from build123d import *

# Parameters (mm, degrees)
BOSS_EXTRUDE1_DEPTH = 5.75
SKETCH2_R           = 2.5
BOSS_EXTRUDE2_DEPTH = 10.5
BOSS_EXTRUDE3_DEPTH = 16.25
SKETCH4_R           = 5
SKETCH4_R_2         = 2.5
BOSS_EXTRUDE5_DEPTH = 8.5
SKETCH5_R           = 2.5
BOSS_EXTRUDE6_DEPTH = 16.25
BOSS_EXTRUDE7_START = 8.5
SKETCH6_R           = 5
BOSS_EXTRUDE7_DEPTH = 8.5
BOSS_EXTRUDE8_START = 8
SKETCH7_R           = 2.5
BOSS_EXTRUDE8_DEPTH = 8
SKETCH8_W           = 10.5
SKETCH8_H           = 5
CUT_EXTRUDE2_DEPTH  = 20
SKETCH9_R           = 2.5
BOSS_EXTRUDE9_DEPTH = 22
SKETCH10_R          = 2.5
CUT_EXTRUDE3_DEPTH  = 55
CUT_EXTRUDE4_START  = -22
CUT_EXTRUDE4_DEPTH  = 22
SKETCH12_W          = 1
SKETCH12_H          = 5
CUT_EXTRUDE5_DEPTH  = 10
SKETCH13_W          = 1
SKETCH13_H          = 10.672821352
SKETCH13_H_2        = 10
CUT_EXTRUDE7_DEPTH  = 10


with BuildPart() as part:
    # Sketch1 → Boss-Extrude1 (new body)
    with BuildSketch(Plane.XY):
        with BuildLine():
            ThreePointArc((-5, 0), (0, -5), (5, 0))
            Line((5, 0), (5, 25))
            ThreePointArc((5, 25), (0, 30), (-5, 25))
            Line((-5, 25), (-5, 0))
        make_face()
    extrude(amount=BOSS_EXTRUDE1_DEPTH)

    # Sketch2 → Boss-Extrude2 (add)
    with BuildSketch(Plane.XY.offset(5.75)):
        with Locations(Location((0, 25.008620985, 0), (0, 0, 180))):
            Circle(SKETCH2_R)
    extrude(amount=BOSS_EXTRUDE2_DEPTH)

    # Sketch3 → Boss-Extrude3 (add)
    with BuildSketch(Plane.XY.offset(5.75)):
        with BuildLine():
            Line((5, 0), (5, 25))
            ThreePointArc((5, 25), (0, 30), (-5, 25))
            Line((-5, 25), (-5, 0))
            ThreePointArc((-5, 0), (0, -5), (5, 0))
        make_face()
    extrude(amount=BOSS_EXTRUDE3_DEPTH)

    # Sketch4 → Boss-Extrude5 (add)
    with BuildSketch(Plane.XY.offset(22)):
        Circle(SKETCH4_R)
        Circle(SKETCH4_R_2, mode=Mode.SUBTRACT)
    extrude(amount=BOSS_EXTRUDE5_DEPTH)

    # Sketch5 → Boss-Extrude6 (add)
    with BuildSketch(Plane.XY.offset(22)):
        Circle(SKETCH5_R)
    extrude(amount=BOSS_EXTRUDE6_DEPTH)

    # Sketch6 → Boss-Extrude7 (add)
    with BuildSketch(Plane(origin=(0, 0, 0), x_dir=(-1, 0, 0), z_dir=(0, 0, -1)).offset(BOSS_EXTRUDE7_START)):
        Circle(SKETCH6_R)
    extrude(amount=-BOSS_EXTRUDE7_DEPTH)

    # Sketch7 → Boss-Extrude8 (add)
    with BuildSketch(Plane(origin=(0, 0, -8.5), x_dir=(-1, 0, 0), z_dir=(0, 0, -1)).offset(BOSS_EXTRUDE8_START)):
        with Locations(Location((0, 0, 0), (0, 0, 180))):
            Circle(SKETCH7_R)
    extrude(amount=-BOSS_EXTRUDE8_DEPTH)

    # Sketch8 → Cut-Extrude2 (cut)
    with BuildSketch(Plane.ZY.offset(5)):
        Polygon((16.25, 25), (5.75, 25), (5.75, 7.741676668), (5.75, 7), (16.25, 7), (16.25, 7.741676668), align=None)
        with Locations((11, 27.5)):
            Rectangle(SKETCH8_W, SKETCH8_H)
    extrude(amount=-CUT_EXTRUDE2_DEPTH, mode=Mode.SUBTRACT)

    # Sketch9 → Boss-Extrude9 (add)
    with BuildSketch(Plane.XY.offset(22)):
        with Locations(Location((0, 25, 0), (0, 0, 90))):
            Circle(SKETCH9_R)
    extrude(amount=-BOSS_EXTRUDE9_DEPTH)

    # Sketch10 → Cut-Extrude3 (cut)
    with BuildSketch(Plane(origin=(0, 0, -16.5), x_dir=(-1, 0, 0), z_dir=(0, 0, -1))):
        Circle(SKETCH10_R)
    extrude(amount=-CUT_EXTRUDE3_DEPTH, mode=Mode.SUBTRACT)

    # Sketch11 → Cut-Extrude4 (cut)
    with BuildSketch(Plane(origin=(0, 0, 0), x_dir=(-1, 0, 0), z_dir=(0, 0, -1)).offset(CUT_EXTRUDE4_START)):
        with BuildLine():
            ThreePointArc((-2.5, 25), (0, 22.5), (2.5, 25))
            Line((2.5, 25), (-2.5, 25))
        make_face()
        with BuildLine():
            Line((-2.5, 25), (2.5, 25))
            ThreePointArc((2.5, 25), (0, 27.5), (-2.5, 25))
        make_face()
    extrude(amount=CUT_EXTRUDE4_DEPTH, mode=Mode.SUBTRACT)

    # Sketch12 → Cut-Extrude5 (cut, symmetric)
    with BuildSketch(Plane(origin=(0, 0, 0), x_dir=(0, 0, -1), z_dir=(1, 0, 0))):
        with Locations((8, 2.5)):
            Rectangle(SKETCH12_W, SKETCH12_H)
        with Locations((8, -2.5)):
            Rectangle(SKETCH12_W, SKETCH12_H)
        with Locations((-30, 2.5)):
            Rectangle(SKETCH12_W, SKETCH12_H)
        with Locations((-30, -2.5)):
            Rectangle(SKETCH12_W, SKETCH12_H)
    extrude(amount=CUT_EXTRUDE5_DEPTH, both=True, mode=Mode.SUBTRACT)

    # Sketch13 → Cut-Extrude7 (cut)
    with BuildSketch(Plane(origin=(5, 0, 0), x_dir=(0, 0, -1), z_dir=(1, 0, 0))):
        with Locations((7, 0.336410676)):
            Rectangle(SKETCH13_W, SKETCH13_H)
        with Locations((-29, 0)):
            Rectangle(SKETCH13_W, SKETCH13_H_2)
    extrude(amount=-CUT_EXTRUDE7_DEPTH, mode=Mode.SUBTRACT)


solid = part.part
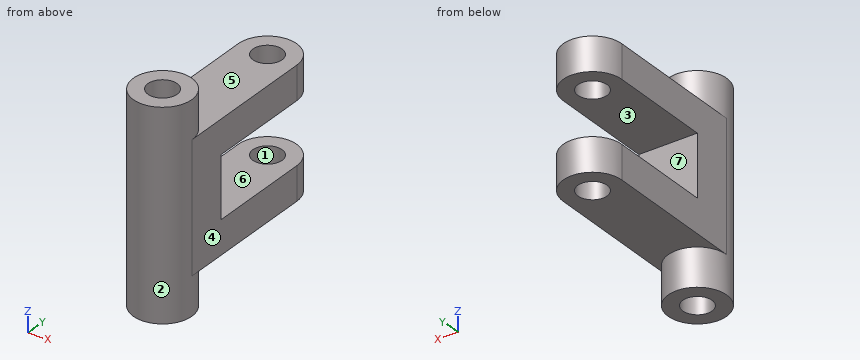
Design review of the part built by this model. Coordinates are the model's own, in mm. Face numbers are marked on the shaded views. A direction names the side the tool comes from. Round coordinates to 2 decimals unless told otherwise and drop trailing zeros. Order: outer loops, then holes, each group sorted by start corner. A loop starts at its lowest first (then second) coordinate and runs counter-clockwise, first axis right, second up. Notation, with made-up numbers: M 19.25,-6.75 L 71.25,-6.75 A31 ccw 71.25,30.25 Z; hole C 51.5,39.25 d7. An arc over 180 degrees is marked long. Answer as CSV lines item,"result". Start each with the question number.
1) Add section A-A (x = 0). Give the boundary of the cut face in (y, z).
2) Add section C-C (y = 3). Give the boundary of the cut face in (x, z).
3) Add section B-B (z = 20.5). Give the boundary of the cut face in (x, y).
4) For pin 1 Ø6 at (x, y) = (0, 25) entering from +Z; pin 2 Ø6 at (x, y) = (0, 25) entering from -Z; pin 3 Ø3 at (x, z) = (-3.5, -1.5) entering from -Y; pin 4 Ø4.5 at (x, y) = (0, 0) entering from +Z, all flat-tipped, find the tip position at first contact; note any pin that passes through.
5) The part is to be moulded in two halves that separate along Z. For the marked faces 4, 5, 6 and 7, say which applies: +Z half, -Z half, draft (parallel to the pull), parting line (faces both ways), or undercut.
6) Tool access review of the marked faces 1, 2 and 3: name each direction out of +Z, -Z, +X, -X, +Y, -Y from which nothing blocks a thin tool from reaching the whole face with its end or side.
7) Wall thickness on line 1 along Y through (x, z) = (0, 19.05); line 2 along Z through (x, y) = (2.25, 16.5); line 3 along Y through (x, z) = (2, 2): over which ranges is each line inside the solid? List them lowest first. Write a range as [from, to].
8) Add section D-D (y = 12). Give the boundary of the cut face in (x, z).
Resolved:
1,outline,"M -5,-6.5 L -2.5,-6.5 L -2.5,28.5 L -5,28.5 Z; M 2.5,-6.5 L 5,-6.5 L 5,0 L 22.5,0 L 22.5,5.75 L 7,5.75 L 7,16.25 L 22.5,16.25 L 22.5,22 L 5,22 L 5,28.5 L 2.5,28.5 Z; M 27.5,0 L 30,0 L 30,5.75 L 27.5,5.75 Z; M 27.5,16.25 L 30,16.25 L 30,22 L 27.5,22 Z"
2,outline,"M -5,0 L -4,0 L -4,-6.5 L 4,-6.5 L 4,0 L 5,0 L 5,22 L 4,22 L 4,28.5 L -4,28.5 L -4,22 L -5,22 Z"
3,outline,"M -5,0 A5 ccw 5,0 L 5,25 A5 ccw -5,25 Z; hole C 0,0 d5; hole C 0,25 d5"
4,pin 1,"z = 22"
4,pin 2,"z = 0"
4,pin 3,"y = -4.58"
4,pin 4,"through"
5,face 4,"draft"
5,face 5,"+Z half"
5,face 6,"undercut"
5,face 7,"undercut"
6,face 1,"+Z, -Z"
6,face 2,"none"
6,face 3,"+X, -X, +Y"
7,line 1,"[-5, -2.5], [2.5, 22.5], [27.5, 30]"
7,line 2,"[0, 5.75], [16.25, 22]"
7,line 3,"[-4.58, -1.5], [1.5, 23.5], [26.5, 29.58]"
8,outline,"M -5,0 L 5,0 L 5,5.75 L -5,5.75 Z; M -5,16.25 L 5,16.25 L 5,22 L -5,22 Z"
